```python
from build123d import *

# Parameters (mm, degrees)
BOSS_EXTRUDE1_DEPTH = 3
SKETCH2_W           = 2.8
SKETCH2_H           = 3
CUT_EXTRUDE1_DEPTH  = 13.389511693


with BuildPart() as part:
    # Sketch1 → Boss-Extrude1 (new body)
    with BuildSketch(Plane(origin=(0, 0, 0), x_dir=(1, 0, 0), z_dir=(0, 1, 0))):
        with BuildLine():
            Line((-8.5, 0), (-8.5, 1))
            Line((-8.5, 1), (8.5, 1))
            Line((8.5, 1), (8.5, 0))
            ThreePointArc((8.5, 0), (0, -8.5), (-8.5, 0))
        make_face()
    extrude(amount=BOSS_EXTRUDE1_DEPTH)

    # Sketch2 → Cut-Extrude1 (cut, through all)
    with BuildSketch(Plane(origin=(0, 3, 0), x_dir=(1, 0, 0), z_dir=(0, 1, 0))):
        with Locations((-4, -0.5)):
            Rectangle(SKETCH2_W, SKETCH2_H)
        with Locations((4, -0.5)):
            Rectangle(SKETCH2_W, SKETCH2_H)
    extrude(amount=-CUT_EXTRUDE1_DEPTH, mode=Mode.SUBTRACT)


solid = part.part
```
Can you work these out from the model? Positions are in its coordinate system, mm. A direction names the side the tool comes from. Coordinates: 2 decimals unless noted, no trailing zeros. Loops run counter-clockwise (first coordinate to the right, second up) from the corner with the lowest first, then second, coordinate; pieces in that order, holes last. Notation, with made-up numbers: (21.25, 67) -> (53.25, 67) arc R37 cw to (53.25, 105) -> close; hole circle Ø2 at (32.25, -12). An arc over 180 degrees is marked (long way). Put each result on its own line as item: value. Start each with the question number.
Q1. I want a section at C-C (z = 6.5). Write out the boundary of the cut face in (x, y).
Q2. I want a section at A-A (y = 0.2). Write out the boundary of the cut face in (x, z).
Q3. Thinking about a two-plate mould opening in X: for faces 3 (the face through (4, 2, 2)), 4 (the face through (7, 1, -1)), 5 (the face through (-8.5, 1.5, -0.5)), 6 (the face through (-2.6, 2, 1)), which applies, pulls with the +X half, pulls with the -X half, needs draft (parallel to the pull), parting line crosses it, or undercut?
Q4. For faces 1 (the face through (0, 3, 4)), 2 (the face through (-4, 2, 2)), which set-ups out of +Z, -Z, +X, -X, +Y, -Y let a thin tool reach every point of the face, with its end or its side?
Q5. I'm going to push a flat-ended pin straight in: P1, Ø0.8, axis at x = 4, y = 1, coming from the -Z side. Where does the tip first touch, or does it pass through?
Q6. If I drill on line 1 (X direction, y = 1.95, z = 0); line 2 (X direction, y = 2.1, z = 1); line 3 (X direction, y = 2.85, z = 7.5), over which ranges is the centre line in solid material (lowest first)? Write a range as [from, to].
Q7. I want a section at B-B (x = -4). Write out the boundary of the cut face in (y, z).
Taken from the geometry:
1. outline: (-5.48, 0) -> (5.48, 0) -> (5.48, 3) -> (-5.48, 3) -> close
2. outline: (-8.5, -1) -> (-5.4, -1) -> (-5.4, 2) -> (-2.6, 2) -> (-2.6, -1) -> (2.6, -1) -> (2.6, 2) -> (5.4, 2) -> (5.4, -1) -> (8.5, -1) -> (8.5, 0) arc R8.5 ccw to (-8.5, 0) -> close
3. face 3: undercut
3. face 4: needs draft
3. face 5: pulls with the -X half
3. face 6: undercut
4. face 1: +Z, -Z, +X, -X, +Y
4. face 2: -Z, +Y, -Y
5. P1: stops at z = 2
6. line 1: x = [-8.5, -5.4], [-2.6, 2.6], [5.4, 8.5]
6. line 2: x = [-8.44, -5.4], [-2.6, 2.6], [5.4, 8.44]
6. line 3: x = [-4, 4]
7. outline: (0, 2) -> (3, 2) -> (3, 7.5) -> (0, 7.5) -> close
